Read the model definition and answer for the solid it produces. Units are mm, in the model's axes. Face numbers are marked on the shaded views. Coordinates: 2 decimals unless noted, no trailing zeros. Loops run counter-clockwise (first coordinate to the right, second up) from the corner with the lowest first, then second, coordinate; pieces in that order, holes last.
Q1. Straight lines are drawn through the part: line 1 (Y direction, x = 8.5, z = 155); line 2 (Y direction, x = 17.75, z = 115); line 3 (Z direction, x = 11.5, y = -547.5). For each, find the intervals that lie inside material, in ascending order.
Q2. Section A-A (x = 11.75) is taken. Give the vertices of the cut face in (y, z), then the cut area to 3 significant figures.
Q3. Section B-B (y = -713.5) is taken. Give the vertices of the cut face in (x, z), then the cut area to 3 significant figures.
Q4. The mould has two halves that part along Y. Classify the marked faces 1 and 2: pulls with the +Y half, pulls with the -Y half, needs draft (parallel to the pull), parting line crosses it, or undercut.
Q5. Section D-D (y = 540) is taken. Give the vertices of the cut face in (x, z).
Q6. Section C-C (z = 121.5) is taken. Give the vertices of the cut face in (x, y).
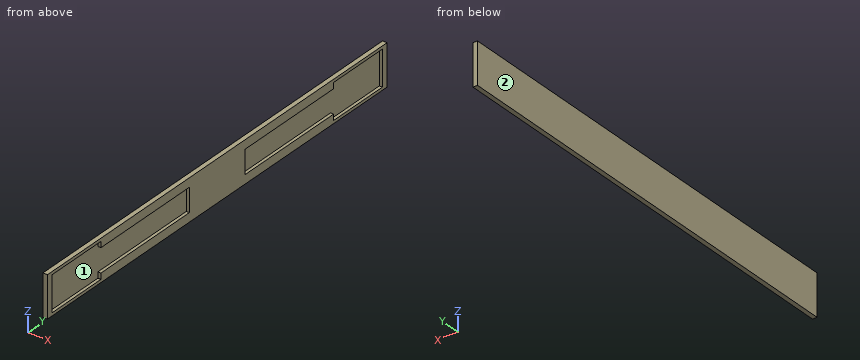
from build123d import *

# Parameters (mm, degrees)
F0_W     = 19.05
F0_H     = 177.8
F1_DEPTH = 927.1
F3_DEPTH = 12.7


with BuildPart() as f1:
    # F0 (on Front) → F1 (new body, symmetric)
    with BuildSketch(Plane.XZ):
        with Locations((9.525, 88.9)):
            Rectangle(F0_W, F0_H)
    extrude(amount=F1_DEPTH, both=True)

    # F2 (on face) → F3 (cut)
    with BuildSketch(Plane.YZ.offset(19.05)):
        Polygon((-901.7, 165.1), (-901.7, 12.7), (-635, 12.7), (-635, 38.1), (-152.4, 38.1), (-152.4, 139.7), (-635, 139.7), (-635, 165.1), align=None)
        Polygon((901.7, 12.7), (901.7, 165.1), (635, 165.1), (635, 139.7), (152.4, 139.7), (152.4, 38.1), (635, 38.1), (635, 12.7), align=None)
    extrude(amount=-F3_DEPTH, mode=Mode.SUBTRACT)


solid = f1.part
Numbers:
1. line 1: y = -927.1 to -901.7, -635 to 635, 901.7 to 927.1
1. line 2: y = -927.1 to -901.7, -152.4 to 152.4, 901.7 to 927.1
1. line 3: z = 0 to 38.1, 139.7 to 177.8
2. outline: (-927.1, 0) - (927.1, 0) - (927.1, 177.8) - (-927.1, 177.8) - close; hole (-901.7, 12.7) - (-635, 12.7) - (-635, 38.1) - (-152.4, 38.1) - (-152.4, 139.7) - (-635, 139.7) - (-635, 165.1) - (-901.7, 165.1) - close; hole (152.4, 38.1) - (635, 38.1) - (635, 12.7) - (901.7, 12.7) - (901.7, 165.1) - (635, 165.1) - (635, 139.7) - (152.4, 139.7) - close
2. area: 150,000 mm2
3. outline: (0, 0) - (19.05, 0) - (19.05, 12.7) - (6.35, 12.7) - (6.35, 165.1) - (19.05, 165.1) - (19.05, 177.8) - (0, 177.8) - close
3. area: 1,450 mm2
4. face 1: undercut
4. face 2: needs draft
5. outline: (0, 0) - (19.05, 0) - (19.05, 38.1) - (6.35, 38.1) - (6.35, 139.7) - (19.05, 139.7) - (19.05, 177.8) - (0, 177.8) - close
6. outline: (0, -927.1) - (19.05, -927.1) - (19.05, -901.7) - (6.35, -901.7) - (6.35, -152.4) - (19.05, -152.4) - (19.05, 152.4) - (6.35, 152.4) - (6.35, 901.7) - (19.05, 901.7) - (19.05, 927.1) - (0, 927.1) - close
